from build123d import *

# Parameters (mm, degrees)
BOSS_EXTRUDE1_DEPTH = 3.175
SKETCH2_W           = 12.7
SKETCH2_H           = 25.4
CUT_EXTRUDE1_DEPTH  = 612.325617511
SKETCH4_W           = 88.9
SKETCH4_H           = 3.175
CUT_EXTRUDE2_DEPTH  = 612.325617511
CUT_EXTRUDE3_DEPTH  = 612.325617511


with BuildPart() as part:
    # Sketch1 → Boss-Extrude1 (new body)
    with BuildSketch(Plane.XY):
        Polygon((0, 0), (190.5, 0), (412.75, -384.948291982), (374.65, -450.939427751), (-184.15, -450.939427751), (-222.25, -384.948291982), align=None)
    extrude(amount=BOSS_EXTRUDE1_DEPTH)

    # Sketch2 → Cut-Extrude1 (cut, through all)
    with BuildSketch(Plane.XY.offset(3.175)):
        with Locations((69.85, -12.7)):
            Rectangle(SKETCH2_W, SKETCH2_H)
        with BuildLine():
            Line((29.329393675, -76.2), (161.170606325, -76.2))
            ThreePointArc((161.170606325, -76.2), (173.870606325, -79.602954744), (183.167651581, -88.9))
            Line((183.167651581, -88.9), (339.952954744, -360.460110958))
            ThreePointArc((339.952954744, -360.460110958), (339.952954744, -385.860110958), (317.955909488, -398.560110958))
            Line((317.955909488, -398.560110958), (-127.455909488, -398.560110958))
            ThreePointArc((-127.455909488, -398.560110958), (-149.452954744, -385.860110958), (-149.452954744, -360.460110958))
            Line((-149.452954744, -360.460110958), (7.332348419, -88.9))
            ThreePointArc((7.332348419, -88.9), (16.629393675, -79.602954744), (29.329393675, -76.2))
        make_face()
        with Locations((120.65, -12.7)):
            Rectangle(SKETCH2_W, SKETCH2_H)
    extrude(amount=-CUT_EXTRUDE1_DEPTH, mode=Mode.SUBTRACT)

    # Sketch4 → Cut-Extrude2 (cut, through all)
    with BuildSketch(Plane.XY.offset(3.175)):
        with Locations((-114.3, -449.351927751)):
            Rectangle(SKETCH4_W, SKETCH4_H)
        with Locations((25.4, -449.351927751)):
            Rectangle(SKETCH4_W, SKETCH4_H)
        with Locations((165.1, -449.351927751)):
            Rectangle(SKETCH4_W, SKETCH4_H)
        with Locations((304.8, -449.351927751)):
            Rectangle(SKETCH4_W, SKETCH4_H)
        Polygon((-215.9, -395.94681461), (-214.525184671, -395.15306461), (-189.125184671, -439.147155122), (-190.5, -439.940905122), align=None)
        Polygon((406.4, -395.94681461), (405.025184671, -395.15306461), (379.625184671, -439.147155122), (381, -439.940905122), align=None)
    extrude(amount=-CUT_EXTRUDE2_DEPTH, mode=Mode.SUBTRACT)

    # Sketch5 → Cut-Extrude3 (cut, through all)
    with BuildSketch(Plane.XY.offset(3.175)):
        Polygon((-209.55, -362.951246726), (-208.175184671, -363.744996726), (-168.487684671, -295.004230301), (-169.8625, -294.210480301), align=None)
        Polygon((-143.087684671, -251.010139788), (-103.400184671, -182.269373363), (-104.775, -181.475623363), (-144.4625, -250.216389788), align=None)
        Polygon((400.05, -362.951246726), (398.675184671, -363.744996726), (358.987684671, -295.004230301), (360.3625, -294.210480301), align=None)
        Polygon((334.9625, -250.216389788), (333.587684671, -251.010139788), (293.900184671, -182.269373363), (295.275, -181.475623363), align=None)
    extrude(amount=-CUT_EXTRUDE3_DEPTH, mode=Mode.SUBTRACT)


solid = part.part
Input: part model. Units: mm. Frame: model coordinates. A direction names the side the tool comes from. Coordinates: 2 decimals unless noted, no trailing zeros. Order: outer loops, then holes, each group sorted by start corner. A loop starts at its lowest first (then second) coordinate and runs counter-clockwise, first axis right, second up. Notation, with made-up numbers: M -28,62 L -18,62 A32 cw -18,98 Z; hole C 21,84.5 d2. An arc over 180 degrees is marked long. Write item = value, one per line. Start each with the question number.
(1) Line query: line 1 along Y through (x, z) = (129.5, 2); line 2 along X through (y, z) = (-23.5, 0.85); line 3 along Y through (x, z) = (111.5, 2.85). Output: solid intervals per line, ascending. Write a range as [from, to].
(2) Section A-A on x = 217. Output: boundary loops of the cut face in (y, z) (3 decimals).
(3) Pull-direction query (X, two-part tool) for faces 3 (the cylindrical face through (16.468, -79.697, 1.61)), 4 (the flat face through (347.485, -271.905, 1.565)), 5 (the flat face through (-53.12, -92.01, 1.57)); classes: released by +X, released by -X, zero draft, split by the parting line, or undercut.
(4) First-contact query: P1, Ø1.6, axis at y = -450, z = 1, coming from the -X side; P2, Ø1.6, axis at y = -449, z = 1.5, coming from the -X side; P3, Ø1.6, axis at y = -449.5, z = 1.5, coming from the +X side. Flat tips, straight axial feed; report the tip coordinate or a pass-through.
(5) Reachability of faces 1 (the cylindrical face through (173.71, -79.51, 1.61)), 2 (the flat face through (-215.989, -374.104, 1.565)) from +Z, -Z, +X, -X, +Y, -Y: full face, straight path, thin tool, end or side. Return the list, or none.
(6) Section B-B on y = -263.5. Output: boundary loops of the cut face in (x, z) (3 decimals).
(7) Section C-C on y = -58. Output: boundary loops of the cut face in (x, z) (3 decimals).
Result set:
q1.line_1 = [-447.76, -398.56], [-76.2, 0]
q1.line_2 = [-13.57, 63.5], [76.2, 114.3], [127, 204.07]
q1.line_3 = [-450.94, -398.56], [-76.2, 0]
q2.outline = M -450.939,0 L -398.56,0 L -398.56,3.175 L -450.939,3.175 Z; M -147.499,0 L -45.899,0 L -45.899,3.175 L -147.499,3.175 Z
q3.face_3 = undercut
q3.face_4 = released by +X
q3.face_5 = released by -X
q4.P1 = -185.15
q4.P2 = -185.73
q4.P3 = 375.94
q5.face_1 = +Z, -Z
q5.face_2 = +Z, -Z, -X, +Y
q6.outline = M -152.132,0 L -93.473,0 L -93.473,3.175 L -152.132,3.175 Z; M 283.973,0 L 342.632,0 L 342.632,3.175 L 283.973,3.175 Z
q7.outline = M -33.486,0 L 223.986,0 L 223.986,3.175 L -33.486,3.175 Z
